Could you check a few things on this model? Use its own coordinates, in mm. Face numbers are marked on the shaded views. A direction names the side the tool comes from. Round coordinates to 2 decimals unless told otherwise and drop trailing zeros. Loops run counter-clockwise (first coordinate to the right, second up) from the corner with the lowest first, then second, coordinate; pieces in that order, holes last. Notation, with made-up numbers: M 43,-23.75 L 94,-23.75 A17 ccw 94,-8.75 Z; hole C 58,63.5 d2. An arc over 180 degrees is marked long. One line per item, written item: value. Start each with the question number.
Q1. I'm going to push flat-ended pins straight in: pin 1 Ø3.5 at (x, y) = (-5, -7.5) entering from +Z; pin 2 Ø3 at (x, y) = (21.5, -6) entering from -Z; pin 3 Ø5 at (y, z) = (-5.5, 19.5) entering from -X. Where does each tip first touch, or does it pass through?
Q2. Which directions (+Z, -Z, +X, -X, +Y, -Y) give clear straight access to the entire face, cutting with the end or side of a thin tool? Please do the marked faces 1, 2, 3, 4 and 5.
Q3. Imagine slicing it at A-A (z = 40.5). Please give me the cut outline in (x, y), then the cut area to 3 significant figures.
Q4. Imagine slicing it at B-B (z = 26). Please give me the cut outline in (x, y).
Q5. Please list where these lines run through material, in increasing order: line 1 along Y through (x, z) = (27.25, 41.91) (3 decimals); line 2 along X through (y, z) = (-6.35, 6.5); line 3 along X through (y, z) = (-6.35, 11.5).
from build123d import *

# Parameters (mm, degrees)
F1_DEPTH  = 12.7
F5_W      = 7.62
F5_H      = 12.7
F6_DEPTH  = 13.97
F8_DEPTH  = 23.876
F9_R      = 6.34999
F10_R     = 5.08
F12_REACH = 53.0526275257
F14_REACH = 53.0526275257
F15_R     = 3.81
F16_DEPTH = 25.4
F17_R     = 1.27


# Not quite as in the source:
# - a fillet or chamfer is up to 0.001 mm smaller than in the source, because OpenCascade refuses the exact size


with BuildPart() as f1:
    # F0 (on Front) → F1 (new body)
    with BuildSketch(Plane.XZ):
        with BuildLine():
            Line((-10.1574255581, 0.381), (0.0040250971, 0.381))
            ThreePointArc((0.0040250971, 0.381), (18.034, 18.034), (36.0639749029, 0.381))
            Line((36.0639749029, 0.381), (46.2254255581, 0.381))
            ThreePointArc((46.2254255581, 0.381), (18.034, 28.194), (-10.1574255581, 0.381))
        make_face()
    extrude(amount=F1_DEPTH)

    # F3 (on offset) → F4 (join, up to the next surface of F1)
    with BuildSketch(Plane.XY.offset(34.29)):
        Polygon((18.034, 0), (0, 0), (0, -12.7), (36.068, -12.7), (36.068, 0), align=None)
    extrude(until=Until.NEXT, dir=(0, 0, -1))

    # F5 (on face) → F6 (join)
    with BuildSketch(Plane.XY.offset(34.29)):
        with Locations((9.906, -6.35)):
            Rectangle(F5_W, F5_H)
        with Locations((26.162, -6.35)):
            Rectangle(F5_W, F5_H)
    extrude(amount=F6_DEPTH)

    # F7 (on face) → F8 (cut, through all)
    with BuildSketch(Plane(origin=(6.096, 0, 0), x_dir=(0, -1, 0), z_dir=(-1, 0, 0))):
        with BuildLine():
            ThreePointArc((6.35, 45.085), (4.1049359697, 39.6649359697), (9.525, 41.91))
            ThreePointArc((9.525, 41.91), (8.5950640303, 44.1550640303), (6.35, 45.085))
        make_face()
    extrude(amount=-F8_DEPTH, mode=Mode.SUBTRACT)

    # F9 (radius 6.35 in the source; OpenCascade refuses exactly that, so slightly less here)
    f9_edges = [f1.edges().sort_by_distance(p)[0] for p in [
        (9.906, -12.7, 48.26),
        (26.162, -12.7, 48.26),
        (9.906, 0, 48.26),
        (26.162, 0, 48.26),
    ]]
    fillet(f9_edges, radius=F9_R)

    # F10
    f10_edges = [f1.edges().sort_by_distance(p)[0] for p in [
        (36.068, -6.35, 34.29),
        (36.068, -6.35, 21.672021),
        (0, -6.35, 34.29),
        (0, -6.35, 21.672021),
    ]]
    fillet(f10_edges, radius=F10_R)

    f12_end = f1.faces().sort_by_distance((-7.8436707665, -6.35, 11.1914159829))[0]
    # F11 (on face) → F12 (cut, up to a face of the model that its end follows)
    with BuildSketch(Plane(origin=(0, 0, 0.381), x_dir=(1, 0, 0), z_dir=(0, 0, -1))):
        with BuildLine():
            ThreePointArc((-3.2479002305, 6.35), (-6.369857112, 7.6431568814), (-5.0767002305, 4.5212))
            ThreePointArc((-5.0767002305, 4.5212), (-3.7835433491, 5.0568431186), (-3.2479002305, 6.35))
        make_face()
    f12_long = extrude(amount=-F12_REACH, mode=Mode.PRIVATE)
    add(split(f12_long, bisect_by=f12_end, keep=Keep.BOTTOM, mode=Mode.PRIVATE), mode=Mode.SUBTRACT)

    f14_end = f1.faces().sort_by_distance((43.9116707665, -6.35, 11.1914159829))[0]
    # F13 (on face) → F14 (cut, up to a face of the model that its end follows)
    with BuildSketch(Plane(origin=(0, 0, 0.381), x_dir=(1, 0, 0), z_dir=(0, 0, -1))):
        with BuildLine():
            ThreePointArc((42.9735002305, 6.35), (39.8515433491, 7.6431568814), (41.1447002305, 4.5212))
            ThreePointArc((41.1447002305, 4.5212), (42.437857112, 5.0568431186), (42.9735002305, 6.35))
        make_face()
    f14_long = extrude(amount=-F14_REACH, mode=Mode.PRIVATE)
    add(split(f14_long, bisect_by=f14_end, keep=Keep.BOTTOM, mode=Mode.PRIVATE), mode=Mode.SUBTRACT)

    # F15 (on face) → F16 (cut)
    with BuildSketch(Plane.XY.offset(34.29)):
        with Locations((-5.0767002305, -6.35)):
            Circle(F15_R)
        with Locations((41.1447002305, -6.35)):
            Circle(F15_R)
    extrude(amount=-F16_DEPTH, mode=Mode.SUBTRACT)

    # F17
    f17_edges = [f1.edges().sort_by_distance(p)[0] for p in [
        (18.034, 0, 18.034),
        (-7.843671, 0, 11.191416),
        (-7.843671, -12.7, 11.191416),
        (43.911671, -12.7, 11.191416),
        (18.034, -12.7, 18.034),
        (43.911671, 0, 11.191416),
        (18.034, -12.7, 34.29),
        (18.034, 0, 34.29),
    ]]
    fillet(f17_edges, radius=F17_R)


solid = f1.part
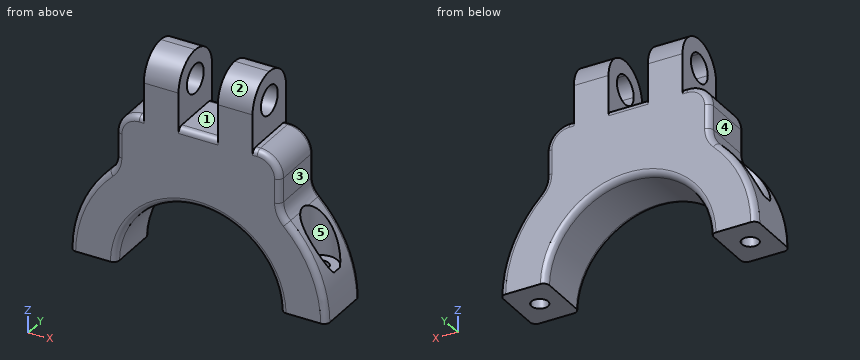
Report:
1. pin 1: stops at z = 8.89
1. pin 2: stops at z = 17.34
1. pin 3: stops at x = -3.05
2. face 1: +Z, +Y, -Y
2. face 2: +Z, +X, -X, -Y
2. face 3: +Z, +X, +Y, -Y
2. face 4: +Z, -X, +Y, -Y
2. face 5: +Z
3. outline: M 6.1,-12.7 L 13.72,-12.7 L 13.72,-9.19 L 6.1,-9.19 Z; M 6.1,-3.51 L 13.72,-3.51 L 13.72,0 L 6.1,0 Z; M 22.35,-12.7 L 29.97,-12.7 L 29.97,-9.19 L 22.35,-9.19 Z; M 22.35,-3.51 L 29.97,-3.51 L 29.97,0 L 22.35,0 Z
3. area: 107 mm²
4. outline: M 0,-11.43 A1.27 ccw 1.27,-12.7 L 34.8,-12.7 A1.27 ccw 36.07,-11.43 L 36.07,-1.27 A1.27 ccw 34.8,0 L 1.27,0 A1.27 ccw 0,-1.27 Z
5. line 1: y = -12.7 to -9.525, -3.175 to 0
5. line 2: x = -9.4 to -6.91, -3.25 to 1.21, 34.86 to 39.32, 42.97 to 45.47
5. line 3: x = -1.27 to 4.14, 31.93 to 37.33
